Model file for the job. Use its own axes, mm. Face numbers are marked on the shaded views. Give positions to 0.01 mm unless a question says otherwise; leave off trailing zeros. Write each loop counter-clockwise with the first axis right and the second up, starting at its lowest first coordinate (ties: lowest second). Pieces come first, ordered by that corner, then holes.
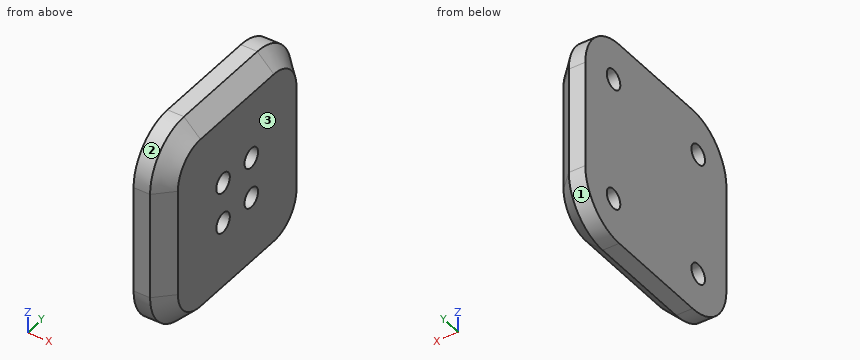
Autodesk Inventor part; units mm, degrees
ref_plane "YZ Plane" through (0, 0, 0) normal (1, 0, 0) x (0, 1, 0)
ref_plane "XZ Plane" through (0, 0, 0) normal (0, 1, 0) x (-1, 0, 0)
ref_plane "XY Plane" through (0, 0, 0) normal (0, 0, 1) x (1, 0, 0)
sketch "草圖1" plane through (0, 0, 0) normal (1, 0, 0) x (0, 1, 0)
  line L0 (-62.5, 62.5) -> (62.5, 62.5)
  line L1 (62.5, 62.5) -> (62.5, -62.5)
  line L2 (62.5, -62.5) -> (-62.5, -62.5)
  line L3 (-62.5, -62.5) -> (-62.5, 62.5)
  line L4 (-62.5, 62.5) -> (62.5, -62.5) construction
  line L5 (62.5, 62.5) -> (-62.5, -62.5) construction
  point P0 (0, 0)
  dimension "d0" = 125
  dimension "d1" = 125
extrude "擠出1" add sketch "草圖1" along normal blind 20
fillet "圓角1" radius 30 4 edges at (10, 62.5, 62.5) (10, -62.5, 62.5) (10, 62.5, -62.5) (10, -62.5, -62.5)
chamfer "倒角1" distance 10 angle 45 8 edges at (20, 0, 62.5) (20, -53.7132, 53.7132) (20, -62.5, 0) (20, -53.7132, -53.7132) (20, 0, -62.5) (20, 53.7132, -53.7132) (20, 62.5, 0) (20, 53.7132, 53.7132)
sketch "草圖2" plane through (20, 0, 0) normal (1, 0, 0) x (0, 0, -1)
  line L0 (-12.5, -12.5) -> (12.5, -12.5)
  line L1 (12.5, -12.5) -> (12.5, 12.5)
  line L2 (12.5, 12.5) -> (-12.5, 12.5)
  line L3 (-12.5, 12.5) -> (-12.5, -12.5)
  line L4 (-12.5, -12.5) -> (12.5, 12.5) construction
  line L5 (12.5, -12.5) -> (-12.5, 12.5) construction
  point P0 (0, 0)
  dimension "d8" = 25
  dimension "d9" = 25
hole "孔1" at (20, 12.5, 12.5) at (20, 12.5, -12.5) at (20, -12.5, 12.5) at (20, -12.5, -12.5) direction (-1, 0, 0) diameter 12 depth 10 tip angle 118
sketch "草圖3" plane through (0, 0, 0) normal (-1, 0, 0) x (0, 0, 1)
  arc A0 (-62.5, -32.5) -> (-32.5, -62.5) centre (-32.5, -32.5) ccw
  line L0 (-32.5, -62.5) -> (32.5, -62.5)
  arc A1 (32.5, -62.5) -> (62.5, -32.5) centre (32.5, -32.5) ccw
  line L1 (62.5, -32.5) -> (62.5, 32.5)
  arc A2 (62.5, 32.5) -> (32.5, 62.5) centre (32.5, 32.5) ccw
  line L2 (32.5, 62.5) -> (-32.5, 62.5)
  arc A3 (-32.5, 62.5) -> (-62.5, 32.5) centre (-32.5, 32.5) ccw
  line L3 (-62.5, 32.5) -> (-62.5, -32.5)
  line L4 (37.5, 37.5) -> (-37.5, 37.5)
  line L5 (-37.5, 37.5) -> (-37.5, -37.5)
  line L6 (-37.5, -37.5) -> (37.5, -37.5)
  line L7 (37.5, -37.5) -> (37.5, 37.5)
  line L8 (37.5, 37.5) -> (-37.5, -37.5) construction
  line L9 (-37.5, 37.5) -> (37.5, -37.5) construction
  point P0 (0, 0)
  dimension "d17" = 75
  dimension "d18" = 75
hole "孔2" at (0, -37.5, 37.5) at (0, -37.5, -37.5) at (0, 37.5, -37.5) at (0, 37.5, 37.5) direction (1, 0, 0) diameter 12 depth 10 tip angle 118
properties part number "exercise3-1-5"
1. Probe probe 1 along Z at (x, y) = (13.25, -12.5); probe 2 along Z at (x, y) = (6, -37.5); probe 3 along Y at (x, z) = (18, -13.5). List the from-to ranges inside material, lowest first.
Calculated:
probe 1: z = -59.25 to -18.5, -6.5 to 6.5, 18.5 to 59.25
probe 2: z = -62.08 to -43.5, -31.5 to 31.5, 43.5 to 62.08
probe 3: y = -54.5 to -18.42, -6.58 to 6.58, 18.42 to 54.5
2. Slice it at A-A, the plane z = 26. Write the cut outline in (x, y), and give its area (3 significant figures).
Calculated:
outline: (0, -62.5) - (10, -62.5) - (20, -52.5) - (20, 52.5) - (10, 62.5) - (0, 62.5) - close
area: 2,400 mm2
3. Pull direction Y, two halves, no side cores. Call the marked faces 1, 2 and 3: +Y half, -Y half, draft (parallel to the pull), parting line (faces both ways), or undercut.
Calculated:
face 1: +Y half
face 2: -Y half
face 3: draft
4. Pin check, flat tips, straight feed: P1, Ø5, axis at x = 15, z = -46.5, coming from the +Y side; P2, Ø2, axis at x = 11.5, z = -10.5, coming from the +Y side; P3, Ø1.5, axis at x = 5.5, y = -41.5, coming from the -Z side. Stop position of each tip, or through.
Calculated:
P1: stops at y = 56.5
P2: stops at y = 62
P3: stops at z = -61.34
